from build123d import *

# Parameters (mm, degrees)
SKETCH1_W               = 55
SKETCH1_H               = 75
BOSS_EXTRUDE1_DEPTH     = 5
SKETCH5_W               = 5
SKETCH5_H               = 30
SKETCH5_W_2             = 15
SKETCH5_H_2             = 5
CUT_EXTRUDE3_DEPTH      = 1
CUT_EXTRUDE3_DEPTH_BACK = 6
SKETCH6_R               = 1.5875
CUT_EXTRUDE4_DEPTH      = 6


with BuildPart() as part:
    # Sketch1 → Boss-Extrude1 (new body)
    with BuildSketch(Plane(origin=(0, 0, 0), x_dir=(1, 0, 0), z_dir=(0, 1, 0))):
        with Locations((27.5, 37.5)):
            Rectangle(SKETCH1_W, SKETCH1_H)
    extrude(amount=BOSS_EXTRUDE1_DEPTH)

    # Sketch5 → Cut-Extrude3 (cut, two sides)
    with BuildSketch(Plane(origin=(0, 5, 0), x_dir=(1, 0, 0), z_dir=(0, 1, 0))) as cut_extrude3_sk:
        with Locations((2.5, 37.5)):
            Rectangle(SKETCH5_W, SKETCH5_H)
        with Locations((27.5, 72.5)):
            Rectangle(SKETCH5_W_2, SKETCH5_H_2)
        with Locations((52.5, 37.5)):
            Rectangle(SKETCH5_W, SKETCH5_H)
        with Locations((27.5, 2.5)):
            Rectangle(SKETCH5_W_2, SKETCH5_H_2)
    extrude(amount=CUT_EXTRUDE3_DEPTH, mode=Mode.SUBTRACT)
    extrude(cut_extrude3_sk.sketch, amount=-CUT_EXTRUDE3_DEPTH_BACK, mode=Mode.SUBTRACT)

    # Sketch6 → Cut-Extrude4 (cut, through all)
    with BuildSketch(Plane(origin=(0, 5, 0), x_dir=(1, 0, 0), z_dir=(0, 1, 0))):
        with Locations((5, 52.5)):
            Circle(SKETCH6_R)
        with Locations((5, 22.5)):
            Circle(SKETCH6_R)
        with Locations((20, 5)):
            Circle(SKETCH6_R)
        with Locations((35, 5)):
            Circle(SKETCH6_R)
        with Locations((50, 22.5)):
            Circle(SKETCH6_R)
        with Locations((50, 52.5)):
            Circle(SKETCH6_R)
        with Locations((35, 70)):
            Circle(SKETCH6_R)
        with Locations((20, 70)):
            Circle(SKETCH6_R)
        with Locations((20, 13.75)):
            Circle(SKETCH6_R)
        with Locations((35, 13.75)):
            Circle(SKETCH6_R)
    extrude(amount=-CUT_EXTRUDE4_DEPTH, mode=Mode.SUBTRACT)


solid = part.part
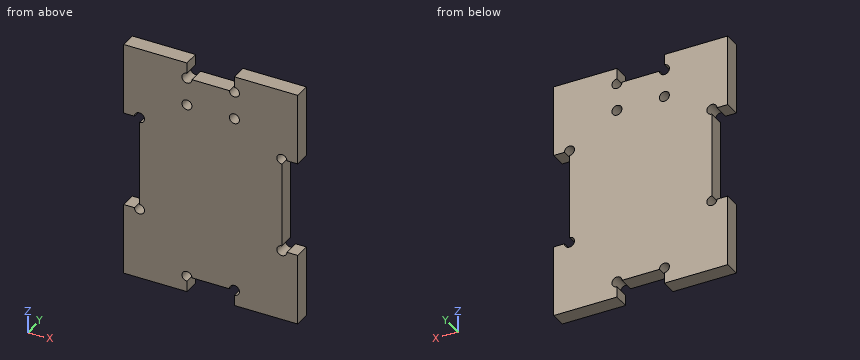
Verification items for the finished model (mm, model axes). Coordinates: 2 decimals unless noted, no trailing zeros. Loops run counter-clockwise (first coordinate to the right, second up) from the corner with the lowest first, then second, coordinate; pieces in that order, holes last. Notation, with made-up numbers: (65, 30) -> (76, 30) arc R7 ccw to (76, 36) -> close; hole circle Ø10 at (20.25, 49.25). An arc over 180 degrees is marked (long way). Answer as CSV lines item,"result".
1) Cross-section at C-C, the plane z = -30. Record the cut outline in (x, y).
Found:
outline,"(5, 0) -> (50, 0) -> (50, 5) -> (5, 5) -> close"
2) Cross-section at B-B, the plane y = 3.05. Count the separate pieces of the cut face and the enclosed holes in it, then the cut area to 3 significant figures.
Found:
separate pieces,"1"
enclosed holes,"2"
area,"3,610 mm2"
3) Cross-section at A-A, the plane z = -13.75. Record the cut outline in (x, y).
Found:
outline,"(0, 0) -> (18.41, 0) -> (18.41, 5) -> (0, 5) -> close; (21.59, 0) -> (33.41, 0) -> (33.41, 5) -> (21.59, 5) -> close; (36.59, 0) -> (55, 0) -> (55, 5) -> (36.59, 5) -> close"
4) Depth check by flat-ended pin: pin 1 (2.5 mm diameter, centred on y = 2.5, z = -32.5, fed in from -X). Enter the tip coordinate at first touch or a pass-through.
Found:
pin 1,"stops at x = 5"
5) Thickness scan on L1, parallel to X at y = 1.9, z = -13.75; L2, parallel to X at y = 1.2, z = -34; L3, parallel to Z at x = 31, y = 1.8. Record the ranges inside material, lowest first. Write a range as from..to.
Found:
L1,"x = 0..18.41, 21.59..33.41, 36.59..55"
L2,"x = 5..50"
L3,"z = -70..-5"
6) Cross-section at D-D, the plane x = 29. Record the cut outline in (y, z), then the cut area to 3 significant figures.
Found:
outline,"(0, -70) -> (5, -70) -> (5, -5) -> (0, -5) -> close"
area,"325 mm2"
